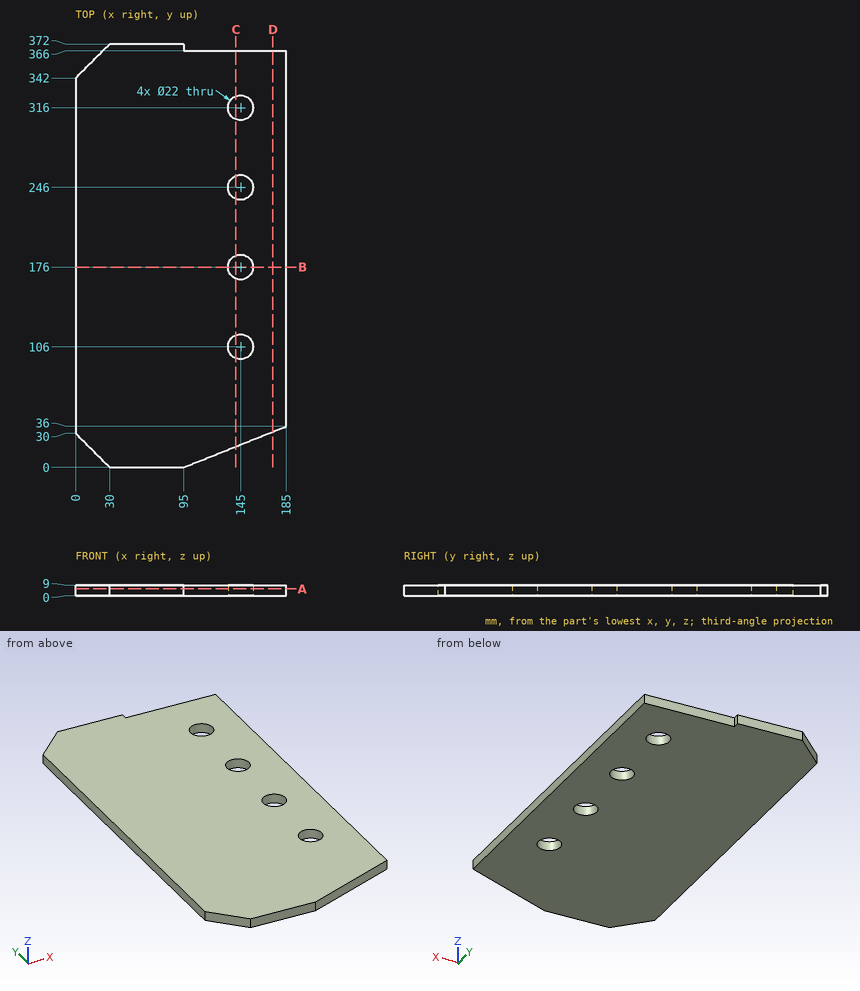
For this review, use the dimensioned drawing (mm, ordinates from the lowest corner) and the shaded views. Coordinates: 2 decimals unless noted, no trailing zeros. Loops run counter-clockwise (first coordinate to the right, second up) from the corner with the lowest first, then second, coordinate; pieces in that order, holes last. Notation, with made-up numbers: (23.25, -4) -> (36.25, -4) arc R33 cw to (36.25, 32) -> close; hole circle Ø9 at (82, 42). An arc over 180 degrees is marked (long way). Use a Markdown table: item, result. Add a question column.
Item 1: We need section D-D, the plane x = 173.5. Write out the cut boundary in (y, z).
Item 2: We need section B-B, the plane y = 176. Write out the cut boundary in (x, z).
Item 3: We need section A-A, the plane z = 6. Write out the cut boundary in (x, y).
Item 4: We need section C-C, the plane x = 141. Write out the cut boundary in (y, z).
Item 5: Clearance check with flat-ended pins moving along their axes: P1, Ø20, axis at x = 145, y = 246, coming from the -Z side; P2, Ø5, axis at x = 112.5, z = 2.5, coming from the -Y side. State where each tip first meets the part, or that it passes through.
Item 6: Wall thickness on L1, parallel to Y at x = 145, z = 6.75; L2, parallel to X at y = 176, z = 5.75; L3, parallel to Y at x = 15, z = 4.75: over which ranges is each line inside the solid? List them lowest first. Write a range as from..to.
Numbers:
| question | item | result |
|---|---|---|
| 1 | outline | (31.4, 0) -> (366, 0) -> (366, 9) -> (31.4, 9) -> close |
| 2 | outline | (0, 0) -> (134, 0) -> (134, 9) -> (0, 9) -> close; (156, 0) -> (185, 0) -> (185, 9) -> (156, 9) -> close |
| 3 | outline | (0, 30) -> (30, 0) -> (95, 0) -> (185, 36) -> (185, 366) -> (95, 366) -> (95, 372) -> (30, 372) -> (0, 342) -> close; hole circle Ø22 at (145, 106); hole circle Ø22 at (145, 176); hole circle Ø22 at (145, 246); hole circle Ø22 at (145, 316) |
| 4 | outline | (18.4, 0) -> (95.75, 0) -> (95.75, 9) -> (18.4, 9) -> close; (116.25, 0) -> (165.75, 0) -> (165.75, 9) -> (116.25, 9) -> close; (186.25, 0) -> (235.75, 0) -> (235.75, 9) -> (186.25, 9) -> close; (256.25, 0) -> (305.75, 0) -> (305.75, 9) -> (256.25, 9) -> close; (326.25, 0) -> (366, 0) -> (366, 9) -> (326.25, 9) -> close |
| 5 | P1 | passes through |
| 5 | P2 | stops at y = 6 |
| 6 | L1 | y = 20..95, 117..165, 187..235, 257..305, 327..366 |
| 6 | L2 | x = 0..134, 156..185 |
| 6 | L3 | y = 15..357 |
